from build123d import *

# Parameters (mm, degrees)
F1_ANGLE = 180
F3_DEPTH = 40


with BuildPart() as f1:
    # F0 (on Front) → F1 (revolve)
    with BuildSketch(Plane.XZ):
        with BuildLine():
            Line((6.25, 20), (-4.25, 20))
            ThreePointArc((-4.25, 20), (-5.664214, 19.414214), (-6.25, 18))
            Line((-6.25, 18), (-6.25, -18))
            ThreePointArc((-6.25, -18), (-5.664214, -19.414214), (-4.25, -20))
            Line((-4.25, -20), (6.25, -20))
            Line((6.25, -20), (6.25, 20))
        make_face()
    revolve(axis=Axis((6.25, 0, 0), (0, 0, -1)), revolution_arc=F1_ANGLE)

    # F2 (on face) → F3 (cut)
    with BuildSketch(Plane.XY.offset(20)):
        with BuildLine():
            Line((-4.25, 0), (16.75, 0))
            ThreePointArc((16.75, 0), (6.25, 10.5), (-4.25, 0))
        make_face()
        with BuildLine():
            ThreePointArc((-4.25, 0), (6.25, -10.5), (16.75, 0))
            Line((16.75, 0), (-4.25, 0))
        make_face()
    extrude(amount=-F3_DEPTH, mode=Mode.SUBTRACT)


with BuildPart() as f4_1:
    # F4: instance of F1
    add(f1.part.mirror(Plane.XZ))


solid = f4_1.part
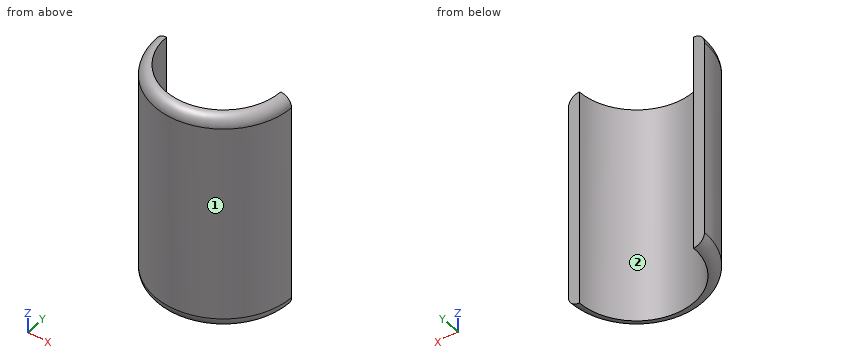
Read the model definition and answer for the solid it produces. Units are mm, in the model's axes. Face numbers are marked on the shaded views. Round coordinates to 2 decimals unless told otherwise and drop trailing zeros. Write each loop counter-clockwise with the first axis right and the second up, starting at its lowest first coordinate (ties: lowest second). Pieces come first, ordered by that corner, then holes. Notation, with made-up numbers: M -23,-7 L 29,-7 A29 cw 29,30 Z; hole C -31,-10 d10. An arc over 180 degrees is marked long. Use a Markdown table: item, result.
1) Straight lines are drawn through the part: line 1 along X through (y, z) = (-0.25, 3.5); line 2 along X through (y, z) = (-7.75, 10.5); line 3 along Y through (x, z) = (6, -0.5). For each, find the intervals that lie inside material, in ascending order. Write a range as [from, to].
Answers follow:
| item | result |
|---|---|
| line 1 | x = [-6.25, -4.25], [16.75, 18.75] |
| line 2 | x = [-3.56, -0.83], [13.33, 16.06] |
| line 3 | y = [-12.5, -10.5] |
2) For a pull along X with two mould halves and no side action, classify the marked faces 1 and 2 as pulls with the +X half, pulls with the -X half, needs draft (parallel to the pull), parting line crosses it, or undercut.
Answers follow:
| item | result |
|---|---|
| face 1 | parting line crosses it |
| face 2 | undercut |
3) The part is cut by section A-A (z = 14). Write down the section's boundary in (x, y).
Answers follow:
| item | result |
|---|---|
| outline | M -6.25,0 A12.5 ccw 18.75,0 L 16.75,0 A10.5 cw -4.25,0 Z |
4) Flat-ended cylindrical pins translate along their axes: pin 1 (1 mm diameter, centred on y = -2, z = 2.5, fed in from +X); pin 2 (2 mm diameter, centred on x = 10.5, z = 12.5, fed in from -Y); pin 3 (5 mm diameter, centred on x = 4.5, z = -10, fed in from +Y); pin 4 (6 mm diameter, centred on x = 2, y = -10, fed in from -Z). Find the tip coordinate at first contact, or state that the pin passes through.
Answers follow:
| item | result |
|---|---|
| pin 1 | stops at x = 18.66 |
| pin 2 | stops at y = -12.07 |
| pin 3 | stops at y = -9.6 |
| pin 4 | stops at z = -20 |
5) The part is cut by section B-B (x = 6.25). Write down the section's boundary in (y, z), plus the area to 3 significant figures.
Answers follow:
| item | result |
|---|---|
| outline | M -12.5,-18 A2 ccw -10.5,-20 L -10.5,20 A2 ccw -12.5,18 Z |
| area | 78.3 mm2 |
